Design review of the part built by this model. Coordinates are the model's own, in mm. A direction names the side the tool comes from. Coordinates: 2 decimals unless noted, no trailing zeros. Loops run counter-clockwise (first coordinate to the right, second up) from the corner with the lowest first, then second, coordinate; pieces in that order, holes last. Notation, with made-up numbers: (-12.5, 58) - (-7.5, 58) arc R19 ccw to (-7.5, 62) - close; hole circle Ø4 at (79.5, 2.25). An arc over 180 degrees is marked (long way). Return JSON: item names as keys, results as strings. Group by question number.
from build123d import *

# Parameters (mm, degrees)
SKETCH1_W           = 75
SKETCH1_H           = 50
BOSS_EXTRUDE1_DEPTH = 2.4
SKETCH2_W           = 69.5
SKETCH2_H           = 44.5
BOSS_EXTRUDE2_DEPTH = 1.8
SKETCH4_R           = 9.6
SKETCH4_R_2         = 14
SKETCH4_R_3         = 2.25
CUT_EXTRUDE1_DEPTH  = 90.866129507
BOSS_EXTRUDE3_DEPTH = 69.5
FILLET1_R           = 3
FILLET2_R           = 3
SKETCH7_R           = 3
CUT_EXTRUDE3_DEPTH  = 2.25
CHAMFER1_SIZE       = 3


with BuildPart() as part:
    # Sketch1 → Boss-Extrude1 (new body)
    with BuildSketch(Plane(origin=(0, 0, 0), x_dir=(1, 0, 0), z_dir=(0, 1, 0))):
        with Locations((36.253665689, 26.173020528)):
            Rectangle(SKETCH1_W, SKETCH1_H)
    extrude(amount=BOSS_EXTRUDE1_DEPTH)

    # Sketch2 → Boss-Extrude2 (add)
    with BuildSketch(Plane(origin=(0, 2.4, 0), x_dir=(1, 0, 0), z_dir=(0, 1, 0))):
        with Locations((36.253665689, 26.173020528)):
            Rectangle(SKETCH2_W, SKETCH2_H)
    extrude(amount=BOSS_EXTRUDE2_DEPTH)

    # Sketch4 → Cut-Extrude1 (cut, through all)
    with BuildSketch(Plane(origin=(0, 0, 0), x_dir=(-1, 0, 0), z_dir=(0, -1, 0))):
        with Locations(Location((-60.718665689, 28.723020528, 0), (0, 0, 90))):
            Circle(SKETCH4_R)
        with Locations(Location((-36.253665689, 28.723020528, 0), (0, 0, 90))):
            Circle(SKETCH4_R_2)
        with Locations(Location((-11.788665689, 28.723020528, 0), (0, 0, 90))):
            Circle(SKETCH4_R)
        with Locations(Location((-67.753665689, 7.173020528, 0), (0, 0, 90))):
            Circle(SKETCH4_R_3)
        with Locations(Location((-4.753665689, 7.180899965, 0), (0, 0, 90))):
            Circle(SKETCH4_R_3)
    extrude(amount=-CUT_EXTRUDE1_DEPTH, mode=Mode.SUBTRACT)

    # Sketch5 → Boss-Extrude3 (add)
    with BuildSketch(Plane(origin=(71.003665689, 0, 0), x_dir=(0, 0, -1), z_dir=(1, 0, 0))):
        Polygon((48.123020528, 4.2), (44.123020528, 4.2), (44.373020528, 8.2), (50.373020528, 8.2), (50.373020528, 7.1), (48.142477117, 4.978263585), align=None)
    extrude(amount=-BOSS_EXTRUDE3_DEPTH)

    # Fillet1
    fillet1_edges = [part.edges().sort_by_distance(p)[0] for p in [
        (-1.246334311, 1.2, -51.173020528),
        (73.753665689, 1.2, -51.173020528),
        (73.753665689, 1.2, -1.173020528),
        (-1.246334311, 1.2, -1.173020528),
    ]]
    fillet(fillet1_edges, radius=FILLET1_R)

    # Fillet2
    # the kernel refuses this fillet: 3 mm, written as the material it takes off along each edge
    with BuildSketch(Plane(origin=(1.753665689, 0, -48.173020528), x_dir=(-1, 0, 0), z_dir=(0, 0, 1))) as fillet2_piece_1:
        with BuildLine():
            CenterArc((0.060612309, -3), FILLET2_R, 11.536959033, 78.463040967)
            Line((3, -2.4), (3.058787754, -2.388))
            ThreePointArc((3.058787754, -2.388), (3.06, -1.2), (3.06, 0))
            Line((3.06, 0), (3, 0.06))
            Line((3, 0.06), (0.060612309, 0.06))
            Line((0.060612309, 0.06), (0.060612309, 0))
        make_face()
    revolve(axis=Axis((1.753665689, 0, -48.173020528), (0, -1, 0)), revolution_arc=90, mode=Mode.SUBTRACT)
    with BuildSketch(Plane(origin=(70.753665689, 0, -51.173020528), x_dir=(0, 0, 1), z_dir=(-1, 0, 0))) as fillet2_piece_2:
        with BuildLine():
            CenterArc((2.939387691, 3), FILLET2_R, 191.536959033, 78.463040967)
            Line((0, 2.4), (-0.058787754, 2.388))
            ThreePointArc((-0.058787754, 2.388), (-0.06, 1.2), (-0.06, 0))
            Line((-0.06, 0), (0, -0.06))
            Line((0, -0.06), (2.939387691, -0.06))
            Line((2.939387691, -0.06), (2.939387691, 0))
        make_face()
    extrude(amount=69, mode=Mode.SUBTRACT)
    with BuildSketch(Plane(origin=(70.753665689, 0, -48.173020528), x_dir=(1, 0, 0), z_dir=(0, 0, 1))) as fillet2_piece_3:
        with BuildLine():
            CenterArc((0.060612309, 3), FILLET2_R, 270, 78.463040967)
            Line((3, 2.4), (3.058787754, 2.388))
            ThreePointArc((3.058787754, 2.388), (3.06, 1.2), (3.06, 0))
            Line((3.06, 0), (3, -0.06))
            Line((3, -0.06), (0.060612309, -0.06))
            Line((0.060612309, -0.06), (0.060612309, 0))
        make_face()
    revolve(axis=Axis((70.753665689, 0, -48.173020528), (0, 1, 0)), revolution_arc=90, mode=Mode.SUBTRACT)
    with BuildSketch(Plane(origin=(73.753665689, 0, -4.173020528), x_dir=(-1, 0, 0), z_dir=(0, 0, -1)), Plane(origin=(-1.246334311, 0, -48.173020528), x_dir=(1, 0, 0), z_dir=(0, 0, 1))) as fillet2_piece_4:
        with BuildLine():
            CenterArc((2.939387691, 3), FILLET2_R, 191.536959033, 78.463040967)
            Line((0, 2.4), (-0.058787754, 2.388))
            ThreePointArc((-0.058787754, 2.388), (-0.06, 1.2), (-0.06, 0))
            Line((-0.06, 0), (0, -0.06))
            Line((0, -0.06), (2.939387691, -0.06))
            Line((2.939387691, -0.06), (2.939387691, 0))
        make_face()
    extrude(amount=44, mode=Mode.SUBTRACT)
    with BuildSketch(Plane(origin=(70.753665689, 0, -4.173020528), x_dir=(0, 0, 1), z_dir=(-1, 0, 0))) as fillet2_piece_5:
        with BuildLine():
            CenterArc((0.060612309, 3), FILLET2_R, 270, 78.463040967)
            Line((3, 2.4), (3.058787754, 2.388))
            ThreePointArc((3.058787754, 2.388), (3.06, 1.2), (3.06, 0))
            Line((3.06, 0), (3, -0.06))
            Line((3, -0.06), (0.060612309, -0.06))
            Line((0.060612309, -0.06), (0.060612309, 0))
        make_face()
    revolve(axis=Axis((70.753665689, 0, -4.173020528), (0, 1, 0)), revolution_arc=90, mode=Mode.SUBTRACT)
    with BuildSketch(Plane(origin=(1.753665689, 0, -1.173020528), x_dir=(0, 1.0, -1.5658770576478976e-12), z_dir=(1, 0, 0))) as fillet2_piece_6:
        with BuildLine():
            CenterArc((3, -2.939387691), FILLET2_R, 101.536959033, 78.463040967)
            Line((0, -2.939387691), (-0.06, -2.939387691))
            Line((-0.06, -2.939387691), (-0.06, 0))
            Line((-0.06, 0), (0, 0.06))
            ThreePointArc((0, 0.06), (1.2, 0.06), (2.388, 0.058787754))
            Line((2.388, 0.058787754), (2.4, 0))
        make_face()
    extrude(amount=69, mode=Mode.SUBTRACT)
    with BuildSketch(Plane(origin=(1.753665689, 0, -4.173020528), x_dir=(0, 0, 1), z_dir=(1, 0, 0))) as fillet2_piece_7:
        with BuildLine():
            CenterArc((0.060612309, -3), FILLET2_R, 11.536959033, 78.463040967)
            Line((3, -2.4), (3.058787754, -2.388))
            ThreePointArc((3.058787754, -2.388), (3.06, -1.2), (3.06, 0))
            Line((3.06, 0), (3, 0.06))
            Line((3, 0.06), (0.060612309, 0.06))
            Line((0.060612309, 0.06), (0.060612309, 0))
        make_face()
    revolve(axis=Axis((1.753665689, 0, -4.173020528), (0, -1, 0)), revolution_arc=90, mode=Mode.SUBTRACT)

    # Sketch7 → Cut-Extrude3 (cut)
    with BuildSketch(Plane.XZ):
        with Locations(Location((4.753665689, -7.180899965, 0), (0, 0, 270))):
            Circle(SKETCH7_R)
        with Locations(Location((67.753665689, -7.173020528, 0), (0, 0, 270))):
            Circle(SKETCH7_R)
    extrude(amount=-CUT_EXTRUDE3_DEPTH, mode=Mode.SUBTRACT)

    # Chamfer1
    # the kernel refuses this chamfer: 3 mm, written as the material it takes off along each edge
    with BuildSketch(Plane(origin=(11.788665689, 4.2, -28.723020528), x_dir=(0, 0, -1), z_dir=(-1, 0, 0))) as chamfer1_piece_1:
        Polygon((9.6 + CHAMFER1_SIZE, 0), (9.6, CHAMFER1_SIZE), (9.6, 0), align=None)
    revolve(axis=Axis((11.788665689, 4.2, -28.723020528), (0, -1, 0)), mode=Mode.SUBTRACT)
    with BuildSketch(Plane(origin=(36.253665689, 4.2, -28.723020528), x_dir=(0, 0, -1), z_dir=(-1, 0, 0))) as chamfer1_piece_2_section:
        Polygon((14 + CHAMFER1_SIZE, 0), (14, CHAMFER1_SIZE), (14, 0), align=None)
    chamfer1_piece_2 = revolve(axis=Axis((36.253665689, 4.2, -28.723020528), (0, -1, 0)), mode=Mode.PRIVATE)
    chamfer1_piece_2 = split(chamfer1_piece_2, bisect_by=Plane(origin=(36.253665689, 0.839630842, -43.912997455), z_dir=(0, 0.06237828615517877, 0.9980525784828888)), keep=Keep.TOP, mode=Mode.PRIVATE)
    add(chamfer1_piece_2, mode=Mode.SUBTRACT)
    with BuildSketch(Plane(origin=(60.718665689, 4.2, -28.723020528), x_dir=(0, 0, -1), z_dir=(-1, 0, 0))) as chamfer1_piece_3:
        Polygon((9.6 + CHAMFER1_SIZE, 0), (9.6, CHAMFER1_SIZE), (9.6, 0), align=None)
    revolve(axis=Axis((60.718665689, 4.2, -28.723020528), (0, -1, 0)), mode=Mode.SUBTRACT)


solid = part.part
Item 1: Add section B-B (z = -29). Give the number of separate pieces and of enclosed holes in the cut face, then the cut area to 3 significant figures.
Item 2: Add section A-A (z = -46). State the section outline as (x, y) points.
Item 3: To check wall thickness, follow line 1 (X direction, y = 2, z = -5); line 2 (X direction, y = 3, z = -21.5); line 3 (Y direction, x = 60, z = -42). State the ranges of each line that lie inside material, in increasing order. Write a range as from..to.
Item 4: For faces 1 (the face through (36, 2.4, -49)), 2 (the face through (15, 4.2, -42)), 3 (the face through (1.504, 3, -15)), 4 (the face through (70, 2.25, -6)), list the 3-axis set-ups (+Z, -Z, +X, -X, +Y, -Y) from which the entire face can be reached by the end or side of a thin tool; tool diameter is ignored.
Item 5: For P1, Ø3.5, axis at x = 67.75, z = -7.17, coming from the -Y side; P2, Ø4.5, axis at y = 5, z = -37, coming from the -X side; P3, Ø8, axis at x = 9.5, z = -18, coming from the +Y side; P4, Ø1.5, axis at y = 1.5, z = -18.5, coming from the +X side, all flat-tipped, find the tip position at first contact; note any pin that passes through.
Item 6: Draft analysis for pull direction Z (two halves, no side actions). For faces 5 (the face through (64.825, 1.109, -6.523)), 6 (the face through (1.825, 1.109, -6.531)), 7 (the face through (36, 3, -48.423)), 8 (the face through (28, 0, -17)), state which applies: pulls with the +Z half, pulls with the -Z half, needs draft (parallel to the pull), parting line crosses it, or undercut.
Answers below:
{
 "1": {"separate pieces": "4", "enclosed holes": "0", "area": "14.0 mm^2"},
 "2": {"outline": "(-1.25, 2.4) arc R3 ccw to (1.69, 0) - (70.81, 0) arc R3 ccw to (73.75, 2.4) - (71, 2.4) - (71, 8.2) - (1.5, 8.2) - (1.5, 2.4) - close"},
 "3": {"line 1": "x = -1.14..2.69, 6.81..65.69, 69.82..73.64", "line 2": "x = 1.5..2.97, 20.61..22.2, 50.31..51.9, 69.54..71", "line 3": "y = 0..4.2"},
 "4": {"face 1": "none", "face 2": "+Z, +X, -X, +Y", "face 3": "+Z, -Z, -X, +Y", "face 4": "-Y"},
 "5": {"P1": "passes through", "P2": "stops at x = 1.5", "P3": "stops at y = 4.2", "P4": "stops at x = 73.72"},
 "6": {"face 5": "undercut", "face 6": "undercut", "face 7": "pulls with the -Z half", "face 8": "needs draft"}
}
